Here's how the part is built. I have some questions about the finished solid (model axes, mm). A direction names the side the tool comes from. Round coordinates to 2 decimals unless told otherwise and drop trailing zeros. Write each loop counter-clockwise with the first axis right and the second up, starting at its lowest first coordinate (ties: lowest second). Pieces come first, ordered by that corner, then holes. Notation, with made-up numbers: M -36,-30 L 20,-30 A17 cw 20,1 Z; hole C -18,-6.75 d3. An arc over 180 degrees is marked long. Use one line per item in the form item = value. Start each with the question number.
Q1. For faces 4 (the face through (0, -35, 42.9)), 5 (the face through (-12.137, -33.349, 49.258)), 6 (the face through (12.1, -33.3, 49)), which set-ups out of +Z, -Z, +X, -X, +Y, -Y let a thin tool reach every point of the face, with its end or its side?
Q2. I want a section at A-A on z = 15.5. List the corners of the cut face in (x, y) for me (3 decimals).
Q3. I'm going to push flat-ended pins straight in: pin 1 Ø1 at (x, z) = (-7, 13) entering from +Y; pin 2 Ø10 at (y, z) = (11.5, 48) entering from +X; pin 3 Ø2 at (x, z) = (21.5, 39.5) entering from +Y. Where does each tip first touch, or does it pass through?
Q4. I need wall thicknesses on line 1 along X through (y, z) = (0, 46); line 2 along X through (y, z) = (-33.3, 50.9); line 3 along Z through (x, y) = (-19.5, 16). Which ranges of each line are inside material? Lowest first, please. Write a range as from..to.
Q5. I want a section at B-B on y = 0. List the corners of the cut face in (x, z) for me.
Q6. We'd pull the mould along Z, two halves only. Please class faces 1 (the face through (-0.242, -33.349, 42.904)), 2 (the face through (24.356, 24.821, 26.08)), 3 (the face through (-8, 33, 52.9)): +Z half, -Z half, draft (parallel to the pull), parting line (faces both ways), or undercut.
Autodesk Inventor part; units mm, degrees
ref_plane "YZ Plane" through (0, 0, 0) normal (1, 0, 0) x (0, 1, 0)
ref_plane "XZ Plane" through (0, 0, 0) normal (0, 1, 0) x (-1, 0, 0)
ref_plane "XY Plane" through (0, 0, 0) normal (0, 0, 1) x (1, 0, 0)
sketch "Sketch1" plane through (0, 0, 0) normal (0, 0, 1) x (1, 0, 0)
  circle A0 centre (0, 0) radius 11.25
  circle A1 centre (0, 0) radius 35.025
  circle A2 centre (0, 0) radius 37.030393
  arc A3 (-32.79294, -17.200962) -> (-31.29294, -19.799038) centre (0, 0) ccw
  line L0 (-32.79294, -17.200962) -> (-31.05471, -16.197395)
  line L1 (-32.79294, -17.200962) -> (-31.05471, -16.197395)
  line L2 (-29.55471, -18.795471) -> (-31.29294, -19.799038)
  line L3 (-31.29294, -19.799038) -> (-29.55471, -18.795471)
  line L4 (-16.197395, -31.05471) -> (-17.200962, -32.79294)
  line L5 (-17.200962, -32.79294) -> (-16.197395, -31.05471)
  arc A4 (-19.799038, -31.29294) -> (-17.200962, -32.79294) centre (0, 0) ccw
  line L6 (-19.799038, -31.29294) -> (-18.795471, -29.55471)
  line L7 (-19.799038, -31.29294) -> (-18.795471, -29.55471)
  arc A5 (17.200962, -32.79294) -> (19.799038, -31.29294) centre (0, 0) ccw
  line L8 (17.200962, -32.79294) -> (16.197395, -31.05471)
  line L9 (17.200962, -32.79294) -> (16.197395, -31.05471)
  line L10 (18.795471, -29.55471) -> (19.799038, -31.29294)
  line L11 (19.799038, -31.29294) -> (18.795471, -29.55471)
  arc A6 (31.29294, -19.799038) -> (32.79294, -17.200962) centre (0, 0) ccw
  line L12 (31.29294, -19.799038) -> (29.55471, -18.795471)
  line L13 (31.05471, -16.197395) -> (32.79294, -17.200962)
  line L14 (32.79294, -17.200962) -> (31.05471, -16.197395)
  line L15 (32.79294, 17.200962) -> (31.05471, 16.197395)
  line L16 (32.79294, 17.200962) -> (31.05471, 16.197395)
  arc A7 (32.79294, 17.200962) -> (31.29294, 19.799038) centre (0, 0) ccw
  line L17 (29.55471, 18.795471) -> (31.29294, 19.799038)
  line L18 (31.29294, 19.799038) -> (29.55471, 18.795471)
  line L19 (16.197395, 31.05471) -> (17.200962, 32.79294)
  line L20 (17.200962, 32.79294) -> (16.197395, 31.05471)
  line L21 (19.799038, 31.29294) -> (18.795471, 29.55471)
  line L22 (19.799038, 31.29294) -> (18.795471, 29.55471)
  line L23 (-17.200962, 32.79294) -> (-16.197395, 31.05471)
  line L24 (-17.200962, 32.79294) -> (-16.197395, 31.05471)
  line L25 (-18.795471, 29.55471) -> (-19.799038, 31.29294)
  line L26 (-19.799038, 31.29294) -> (-18.795471, 29.55471)
  arc A8 (-31.29294, 19.799038) -> (-32.79294, 17.200962) centre (0, 0) ccw
  line L27 (-31.29294, 19.799038) -> (-29.55471, 18.795471)
  line L28 (-31.29294, 19.799038) -> (-29.55471, 18.795471)
  line L29 (-31.05471, 16.197395) -> (-32.79294, 17.200962)
  line L30 (-32.79294, 17.200962) -> (-31.05471, 16.197395)
  arc A9 (-34.800207, -3.961848) -> (-34.800207, 3.961848) centre (-31.75, 0) ccw
  circle A10 centre (-31.75, 0) radius 5
  arc A11 (-3.961848, 34.800207) -> (3.961848, 34.800207) centre (0, 31.75) ccw
  circle A12 centre (0, 31.75) radius 5
  circle A13 centre (31.75, 0) radius 5
  circle A14 centre (31.75, 0) radius 5
  arc A15 (-3.961848, -34.800207) -> (3.961848, -34.800207) centre (0, -31.75) ccw
  circle A16 centre (0, -31.75) radius 5
  circle A17 centre (0, 31.75) radius 4.75
  circle A18 centre (-31.75, 0) radius 4.75
  circle A19 centre (0, -31.75) radius 4.75
  circle A20 centre (31.75, 0) radius 4.75
  circle A21 centre (0, 0) radius 34.775
  circle A22 centre (0, 0) radius 36.75
  point P0 (0, 0)
  point P1 (0, 49.75)
  point P2 (34.563789, -3.82689)
  point P3 (34.563789, 3.82689)
  point P4 (3.82689, 34.563789)
  point P5 (-3.82689, 34.563789)
  point P6 (-34.563789, 3.82689)
  point P7 (-34.563789, -3.82689)
  point P8 (-3.82689, -34.563789)
  point P9 (3.82689, -34.563789)
  dimension "d6" = 70.05
  dimension "d8" = 74.06079
  dimension "d0" = 10
  dimension "d1" = 0.25
  dimension "d4" = 360
  dimension "d7" = 0.25
  dimension "d9" = 73.5
sketch "Sketch1 outline for Extrusion1" plane through (0, 0, 0) normal (0, 0, 1) x (1, 0, 0)
  arc A0 (3.82689, -34.563789) -> (34.563789, -3.82689) centre (0, 0) ccw
  arc A1 (-3.82689, -34.563789) -> (3.82689, -34.563789) centre (0, -31.75) ccw
  arc A2 (-34.563789, -3.82689) -> (-3.82689, -34.563789) centre (0, 0) ccw
  arc A3 (-34.563789, 3.82689) -> (-34.563789, -3.82689) centre (-31.75, 0) ccw
  arc A4 (-3.82689, 34.563789) -> (-34.563789, 3.82689) centre (0, 0) ccw
  arc A5 (3.82689, 34.563789) -> (-3.82689, 34.563789) centre (0, 31.75) ccw
  arc A6 (34.563789, 3.82689) -> (3.82689, 34.563789) centre (0, 0) ccw
  arc A7 (34.563789, -3.82689) -> (34.563789, 3.82689) centre (31.75, 0) ccw
extrude "Extrusion1" add sketch "Sketch1 outline for Extrusion1" along normal blind 52.9
sketch "Skizze4" plane through (0, 0, 52.9) normal (0, 0, 1) x (1, 0, 0)
  circle A0 centre (0, 0) radius 33.79
  dimension "d24" = 67.58
extrude "Extrusion4" cut sketch "Skizze4" against normal blind 10
sketch "Skizze5" plane through (0, 0, 52.9) normal (0, 0, 1) x (1, 0, 0)
  line L0 (-8, -25.79) -> (8, -25.79)
  line L1 (8, -25.79) -> (8, -41.79)
  line L2 (8, -41.79) -> (-8, -41.79)
  line L3 (-8, -41.79) -> (-8, -25.79)
  circle A0 centre (0, 0) radius 33.79
  line L4 (-8, -25.79) -> (8, -41.79) construction
  line L5 (8, -25.79) -> (-8, -41.79) construction
  point P0 (0, -33.79)
  dimension "d27" = 16
  dimension "d28" = 16
extrude "Extrusion5" cut sketch "Skizze5" against normal up to surface (10 mm away) contours L0 L1 A0 L3 | A0 L1 L2 L3 picked at (-0.896461, -28.420935)
ref_plane "Arbeitsebene1" through (-8, -33.84229, 52.9) normal (0, -1, 0) x (0, 0, -1)
sketch "Skizze8" plane through (-8, -33.84229, 52.9) normal (0, -1, 0) x (0, 0, -1)
  circle A0 centre (2, 8) radius 8
  circle A1 centre (2, 8) radius 12.247788
  line L0 (-1.778493, -7.044693) -> (-1.736571, 22.979568)
  line L1 (10, 0) -> (2, 0)
  line L2 (2, 0) -> (2, 8)
  line L3 (2, 8) -> (10, 8)
  line L4 (10, 8) -> (10, 0)
  point P0 (52.9, 8)
  point P1 (3.776106, -5.296677)
  point P2 (-1.741203, 19.662406)
  point P3 (-1.747618, 15.067911)
  point P4 (-1.76734, 0.942582)
  point P5 (-1.773756, -3.651913)
  dimension "d31" = 16
  dimension "d36" = 8
extrude "Extrusion6" add sketch "Skizze8" against normal blind 1 contours L1 L4 A0 L0 A1 | A0 L4 L1
properties part number "2024_08_26_Double_walled_beaker_recess_2,1cm"
Reported:
q1.face_4 = +Z, +X, -X, -Y
q1.face_5 = -X, -Y
q1.face_6 = +X, -Y
q2.outline = M -34.564,-3.827 A34.775 ccw -3.827,-34.564 A4.75 ccw 3.827,-34.564 A34.775 ccw 34.564,-3.827 A4.75 ccw 34.564,3.827 A34.775 ccw 3.827,34.564 A4.75 ccw -3.827,34.564 A34.775 ccw -34.564,3.827 A4.75 ccw Z
q3.pin_1 = 34.16
q3.pin_2 = 34.16
q3.pin_3 = 28.09
q4.line_1 = -36.5..-33.79, 33.79..36.5
q4.line_2 = -12.25..-8, 8..12.25
q4.line_3 = 0..42.9
q5.outline = M -36.5,0 L 36.5,0 L 36.5,52.9 L 33.79,52.9 L 33.79,42.9 L -33.79,42.9 L -33.79,52.9 L -36.5,52.9 Z
q6.face_1 = undercut
q6.face_2 = draft
q6.face_3 = +Z half
